Could you check a few things on this model? Use its own coordinates, in mm. Face numbers are marked on the shaded views. A direction names the side the tool comes from. Give positions to 0.01 mm unless a question says otherwise; leave off trailing zeros. Write each loop counter-clockwise with the first axis right and the second up, starting at its lowest first coordinate (ties: lowest second). Pieces come first, ordered by that corner, then holes. Notation, with made-up numbers: (88.5, 86) -> (119.5, 86) arc R10 ccw to (119.5, 90) -> close; hole circle Ø6 at (-28, 21). An arc over 180 degrees is marked (long way). One line per question, with ' | ' between items.
from build123d import *

# Parameters (mm, degrees)
SKETCH1_W           = 7
SKETCH1_H           = 7
BOSS_EXTRUDE1_DEPTH = 3
FILLET1_R           = 1
SKETCH2_R           = 1
BOSS_EXTRUDE2_DEPTH = 0.2
FILLET2_R           = 1


with BuildPart() as part:
    # Sketch1 → Boss-Extrude1 (new body)
    with BuildSketch(Plane(origin=(0, 0, 0), x_dir=(1, 0, 0), z_dir=(0, 1, 0))):
        Rectangle(SKETCH1_W, SKETCH1_H)
    extrude(amount=BOSS_EXTRUDE1_DEPTH)

    # Fillet1
    fillet1_edges = [part.edges().sort_by_distance(p)[0] for p in [
        (-3.5, 3, 0),
        (0, 3, 3.5),
        (3.5, 3, 0),
        (0, 3, -3.5),
        (3.5, 1.5, 3.5),
        (-3.5, 1.5, 3.5),
        (-3.5, 1.5, -3.5),
        (3.5, 1.5, -3.5),
    ]]
    fillet(fillet1_edges, radius=FILLET1_R)

    # Sketch2 → Boss-Extrude2 (add)
    with BuildSketch(Plane(origin=(0, 3, 0), x_dir=(1, 0, 0), z_dir=(0, 1, 0))):
        with Locations(Location((0, 0, 0), (0, 0, 270))):
            Circle(SKETCH2_R)
    extrude(amount=BOSS_EXTRUDE2_DEPTH)

    # Fillet2
    # the kernel refuses this fillet: 1 mm, written as the material it takes off along each edge
    with BuildSketch(Plane(origin=(0, 3.2, 0), x_dir=(0, 0, 1), z_dir=(-1, 0, 0))) as fillet2_piece_1:
        with BuildLine():
            CenterArc((0.4, -1), FILLET2_R, 53.130102354, 36.869897646)
            Line((0.4, 0), (0.4, 0.02))
            Line((0.4, 0.02), (1, 0.02))
            Line((1, 0.02), (1.02, 0))
            ThreePointArc((1.02, 0), (1.02, -0.1), (1.012, -0.184))
            Line((1.012, -0.184), (1, -0.2))
        make_face()
    revolve(axis=Axis((0, 3.2, 0), (0, 1, 0)), mode=Mode.SUBTRACT)


solid = part.part
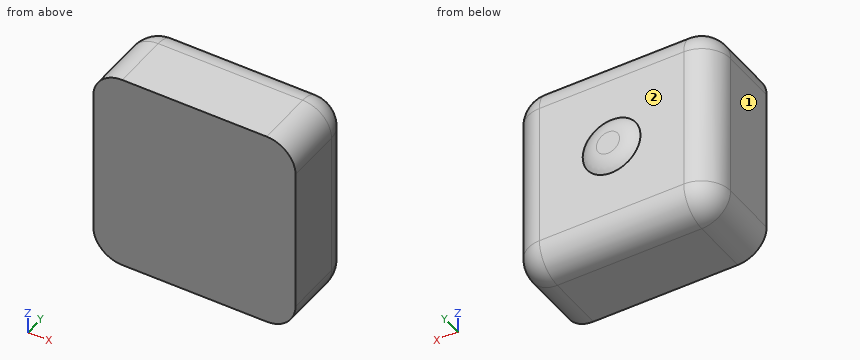
Q1. Will this pin go through, and if not, where does the flat tip stop? pin 1 (2 mm diameter, centred on x = -1.5, z = 0, fed in from +Y) (3 decimals).
Answer below:
pin 1: stops at y = 3.195
Q2. Imagine slicing it at D-D on y = 2.85. Please give me the cut outline in (x, z), and give its area (3 significant figures).
Answer below:
outline: (-3.03, -2.5) arc R0.53 ccw to (-2.5, -3.03) -> (2.5, -3.03) arc R0.53 ccw to (3.03, -2.5) -> (3.03, 2.5) arc R0.53 ccw to (2.5, 3.03) -> (-2.5, 3.03) arc R0.53 ccw to (-3.03, 2.5) -> close | area: 36.4 mm^2
Q3. Imagine slicing it at A-A on y = 1.3. Please give me the cut outline in (x, z).
Answer below:
outline: (-3.5, -2.5) arc R1 ccw to (-2.5, -3.5) -> (2.5, -3.5) arc R1 ccw to (3.5, -2.5) -> (3.5, 2.5) arc R1 ccw to (2.5, 3.5) -> (-2.5, 3.5) arc R1 ccw to (-3.5, 2.5) -> close
Q4. Imagine slicing it at C-C on z = -1.5. Please give me the cut outline in (x, y).
Answer below:
outline: (-3.5, 0) -> (3.5, 0) -> (3.5, 2) arc R1 ccw to (2.5, 3) -> (-2.5, 3) arc R1 ccw to (-3.5, 2) -> close
Q5. On a 3-axis mill with a long thin cutter (end or side, diameter ignored), from which of +Z, -Z, +X, -X, +Y, -Y can I reach the whole of each face in a straight line? I mean the marked faces 1 and 2. Say none if no direction works.
Answer below:
face 1: +Z, -Z, -X, +Y, -Y | face 2: +Y
Q6. If I drill on line 1 along Y through (x, z) = (-0.5, 2.5); line 2 along Z through (x, y) = (2, 2.35); line 3 along Z through (x, y) = (1.25, 2.6), over which ranges is the centre line in solid material (lowest first)?
Answer below:
line 1: y = 0 to 3 | line 2: z = -3.44 to 3.44 | line 3: z = -3.3 to 3.3
Q7. Imagine slicing it at B-B on x = 1.75. Please give me the cut outline in (y, z).
Answer below:
outline: (0, -3.5) -> (2, -3.5) arc R1 ccw to (3, -2.5) -> (3, 2.5) arc R1 ccw to (2, 3.5) -> (0, 3.5) -> close
